Can you work these out from the model? Positions are in its coordinate system, mm. Give positions to 0.01 mm unless a question says otherwise; leave off trailing zeros. Loops run counter-clockwise (first coordinate to the right, second up) from the corner with the lowest first, then second, coordinate; pieces in that order, holes last.
from build123d import *

# Parameters (mm, degrees)
F0_R     = 50.8
F1_DEPTH = 81.28


with BuildPart() as f1:
    # F0 (on Top) → F1 (new body)
    with BuildSketch(Plane.XY):
        Polygon((88.161778, 52.584354), (-1.458498, 102.642516), (-89.620275, 50.058162), (-88.161778, -52.584354), (1.458498, -102.642516), (89.620275, -50.058162), align=None)
        Circle(F0_R, mode=Mode.SUBTRACT)
    extrude(amount=F1_DEPTH)

    # F2 (on Front) → F3 (revolve, cut)
    with BuildSketch(Plane.XZ):
        Polygon((161.132823, 41.287788), (157.832084, 81.28), (89.620275, 81.28), (160.01082, 40.64), align=None)
        Polygon((161.245103, 41.352613), (161.132823, 41.287788), (161.186287, 40.64), align=None)
        Polygon((161.132823, 39.992212), (160.01082, 40.64), (89.620275, 0), (157.832084, 0), align=None)
        Polygon((161.245103, 39.927387), (161.186287, 40.64), (161.132823, 39.992212), align=None)
    revolve(axis=Axis((0, 0, 40.64), (0, 0, 1)), mode=Mode.SUBTRACT)


solid = f1.part
(1) Suppose I cut it at A-A on z = 23. List the corners of the cut face in (x, y) for me.
Returned:
outline: (-89.62, 50.06) - (-88.16, -52.58) - (1.46, -102.64) - (89.62, -50.06) - (88.16, 52.58) - (-1.46, 102.64) - close; hole circle Ø101.6 at (0, 0)
(2) Please list where these lines run through material, in increasing order: probe 1 along X at (y, z) = (27.5, 51.5); probe 2 along Y at (x, z) = (0, 63); probe 3 along X at (y, z) = (16.5, 33.5).
Returned:
probe 1: x = -89.3 to -42.71, 42.71 to 88.52
probe 2: y = -101.83 to -50.8, 50.8 to 101.83
probe 3: x = -89.14 to -48.05, 48.05 to 88.67
(3) Thinking about a two-plate mould opening in X: for faces 1 (the conical face through (-80.263, -47.271, 2.037)), 2 (the conical face through (-0.81, 93.15, 2.04)), 3 (the conical face through (80.263, 47.271, 2.037)), 4 (the cylindrical face through (-11.012, -49.592, 40.071)), which applies, pulls with the +X half, pulls with the -X half, needs draft (parallel to the pull), parting line crosses it, or undercut?
Returned:
face 1: pulls with the -X half
face 2: parting line crosses it
face 3: pulls with the +X half
face 4: undercut
(4) Will these pins go through, and if not, where does the flat tip stop? P1, Ø2, axis at x = -26, z = 31, coming from the -Y side; P2, Ø1.5, axis at x = 55, z = 39, coming from the -Y side; P3, Ø5, axis at x = -25.5, z = 63, coming from the +Y side.
Returned:
P1: stops at y = -87.86
P2: stops at y = -71.15
P3: stops at y = 89.79
(5) Suppose I cut it at C-C on x = -40. List the corners of the cut face in (y, z) for me, plus the area to 3 significant figures.
Returned:
outline: (-79.49, 0) - (-31.32, 0) - (-31.32, 81.28) - (-79.49, 81.28) - close; (31.32, 0) - (79.65, 0) - (79.65, 81.28) - (31.32, 81.28) - close
area: 7,840 mm2
(6) Suppose I cut it at B-B on y = 0. List the corners of the cut face in (x, z) for me.
Returned:
outline: (-88.91, 0) - (-50.8, 0) - (-50.8, 81.28) - (-88.91, 81.28) - close; (50.8, 0) - (88.91, 0) - (88.91, 81.28) - (50.8, 81.28) - close
